Autodesk Inventor part; units mm, degrees
ref_plane "YZ Plane" through (0, 0, 0) normal (1, 0, 0) x (0, 1, 0)
ref_plane "XZ Plane" through (0, 0, 0) normal (0, 1, 0) x (-1, 0, 0)
ref_plane "XY Plane" through (0, 0, 0) normal (0, 0, 1) x (1, 0, 0)
sketch "Sketch1" plane through (0, 0, 0) normal (0, 1, 0) x (-1, 0, 0)
  line L0 (173, 61.75) -> (-173, 61.75)
  line L1 (-173, 61.75) -> (-173, -61.75)
  line L2 (-173, -61.75) -> (173, -61.75)
  line L3 (173, -61.75) -> (173, 61.75)
  point P0 (0, 0)
  point P1 (0, -61.75)
  point P2 (173, 0)
  dimension "d0" = 346
  dimension "d1" = 123.5
extrude "Extrusion1" add sketch "Sketch1" along normal blind 4
sketch "Esboço2" plane through (0, 4, 0) normal (0, 1, 0) x (1, 0, 0)
  line L0 (173, 61.75) -> (-173, 61.75)
  line L1 (118.5, 61.75) -> (70.5, 61.75)
  line L2 (70.5, 61.75) -> (70.5, 57.75)
  line L3 (70.5, 57.75) -> (118.5, 57.75)
  line L4 (118.5, 57.75) -> (118.5, 61.75)
  line L5 (173, -61.75) -> (173, 61.75)
  line L6 (24, 61.75) -> (-24, 61.75)
  line L7 (-24, 61.75) -> (-24, 57.75)
  line L8 (-24, 57.75) -> (24, 57.75)
  line L9 (24, 57.75) -> (24, 61.75)
  line L10 (-70.5, 61.75) -> (-118.5, 61.75)
  line L11 (-118.5, 61.75) -> (-118.5, 57.75)
  line L12 (-118.5, 57.75) -> (-70.5, 57.75)
  line L13 (-70.5, 57.75) -> (-70.5, 61.75)
  circle A0 centre (24, 57.75) radius 1
  circle A1 centre (70.5, 57.75) radius 1
  circle A2 centre (-24, 57.75) radius 1
  circle A3 centre (-70.5, 57.75) radius 1
  circle A4 centre (-118.5, 57.75) radius 1
  circle A5 centre (118.5, 57.75) radius 1
  point P0 (0, 0)
  dimension "d4" = 48
  dimension "d5" = 4
  dimension "d6" = 54.5
  dimension "d7" = 48
  dimension "d8" = 46.5
  dimension "d9" = 48
  dimension "d10" = 46.5
  dimension "d11" = 2
  dimension "d12" = 2
  dimension "d13" = 2
  dimension "d14" = 2
  dimension "d15" = 2
  dimension "d16" = 2
extrude "Extrusão2" cut sketch "Esboço2" against normal blind 10
mirror "Espelhamento1" about plane through (0, 0, 0) normal (0, 0, 1) of "Extrusão2"
sketch "Esboço3" plane through (0, 4, 0) normal (0, 1, 0) x (1, 0, 0)
  line L0 (-118.5, 61.75) -> (-173, 61.75)
  line L1 (-173, 61.75) -> (-165, 61.75)
  line L2 (-165, 61.75) -> (-165, 21.75)
  line L3 (-165, 21.75) -> (-173, 21.75)
  line L4 (-173, 21.75) -> (-173, 61.75)
  line L5 (-173, 61.75) -> (-173, -61.75)
  line L6 (-173, -61.75) -> (-165, -61.75)
  line L7 (-165, -61.75) -> (-165, -21.75)
  line L8 (-165, -21.75) -> (-173, -21.75)
  line L9 (-173, -21.75) -> (-173, -61.75)
  circle A0 centre (-165, 21.75) radius 1
  circle A1 centre (-165, -21.75) radius 1
  point P0 (0, 0)
  dimension "d19" = 8
  dimension "d20" = 40
  dimension "d21" = 40
  dimension "d22" = 43.5
  dimension "d23" = 2
  dimension "d24" = 2
extrude "Extrusão3" cut sketch "Esboço3" against normal blind 10
mirror "Espelhamento2" about plane through (0, 0, 0) normal (1, 0, 0) of "Extrusão3"
properties part number "fechamento superior"
Verification items for the finished model (mm, model axes). Coordinates: 2 decimals unless noted, no trailing zeros. Order: outer loops, then holes, each group sorted by start corner. A loop starts at its lowest first (then second) coordinate and runs counter-clockwise, first axis right, second up. Notation, with made-up numbers: M -28,87 L 10,87 A11 cw 10,93 Z; hole C -23.5,56 d6. An arc over 180 degrees is marked long. Write each question's results on one line, items separated by ' | '.
1) Scan lines: line 1 along X through (y, z) = (2.25, -41); line 2 along Z through (x, y) = (-104, 3.5). Record each from-to range of solid material in increasing order. Write a range as [from, to].
Solved:
line 1: x = [-165, 165] | line 2: z = [-57.75, 57.75]
2) Section check B-B on x = -98.5. Record the cut outline in (y, z), plus the area to 3 significant figures.
Solved:
outline: M 0,-57.75 L 4,-57.75 L 4,57.75 L 0,57.75 Z | area: 462 mm²
3) Gauge pin test, flat ends, axial feed: pin 1 Ø2 at (x, y) = (-88, 2.5) entering from +Z; pin 2 Ø1.2 at (x, z) = (118.5, 57.75) entering from +Y; pin 3 Ø2 at (y, z) = (1.5, -41) entering from -X; pin 4 Ø6 at (x, z) = (-105, -30.5) entering from -Y. Record the tip position at first contact, or that the pin passes through.
Solved:
pin 1: stops at z = 57.75 | pin 2: passes through | pin 3: stops at x = -165 | pin 4: stops at y = 0
4) Section check A-A on z = -29. Record the cut outline in (x, y), plus the area to 3 significant figures.
Solved:
outline: M -165,0 L 165,0 L 165,4 L -165,4 Z | area: 1,320 mm²
